Read the model definition and answer for the solid it produces. Units are mm, in the model's axes. Face numbers are marked on the shaded views. Give positions to 0.01 mm unless a question says otherwise; leave off trailing zeros. Loops run counter-clockwise (first coordinate to the right, second up) from the corner with the lowest first, then second, coordinate; pieces in that order, holes last. Notation, with made-up numbers: (20.25, 18.25) -> (66.25, 18.25) arc R12 cw to (66.25, 31.25) -> close; hole circle Ø11 at (3.5, 25). An arc over 180 degrees is marked (long way). One line per item, written item: value. Start each with the question number.
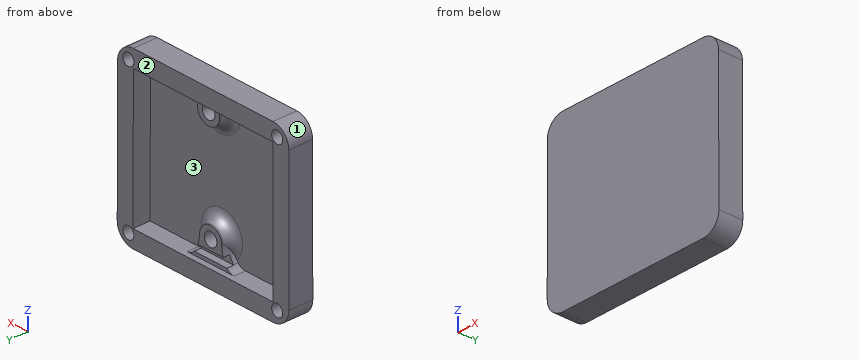
from build123d import *

# Parameters (mm, degrees)
CROQUIS1_R              = 1.3
SALIENTE_EXTRUIR1_DEPTH = 5
VACIADO1_START          = -5
VACIADO1_DEPTH          = 5
VACIADO1_2_OUTLINE_R    = 1.3
VACIADO1_2_DEPTH        = 5
VACIADO1_3_OUTLINE_R    = 1.3
VACIADO1_3_DEPTH        = 5
SALIENTE_EXTRUIR2_START = -1.65
CROQUIS2_R              = 3.5
CROQUIS2_R_2            = 2
SALIENTE_EXTRUIR2_DEPTH = 3.35
CROQUIS3_R              = 2
CORTAR_EXTRUIR1_DEPTH   = 5
REDONDEO1_R             = 5
CROQUIS4_R              = 1.75
CORTAR_EXTRUIR2_DEPTH   = 4
REDONDEO2_R             = 3
CROQUIS5_W              = 10.71017297
CROQUIS5_H              = 2.16113269
CORTAR_EXTRUIR3_DEPTH   = 2
REDONDEO3_R             = 5
CROQUIS6_W              = 134.393326308
CROQUIS6_H              = 117.100902836
CORTAR_EXTRUIR4_DEPTH   = 3


# Read off the part's stored shape, not the designer's step: Vaciado1
with BuildPart() as part:
    # Croquis1 → Saliente-Extruir1 (new body)
    with BuildSketch(Plane(origin=(0, 0, 0), x_dir=(1, 0, 0), z_dir=(0, 1, 0))):
        Polygon((-21.910650365, -18.655769069), (22.326249635, -18.714369069), (22.443043136, 20.685314639), (-21.956956864, 20.744230931), align=None)
        with Locations(Location((0.268043136, -16.390769069, 0), (0, 0, 270))):
            Circle(CROQUIS1_R, mode=Mode.SUBTRACT)
        with Locations(Location((-0.366956864, 14.724230931, 0), (0, 0, 270))):
            Circle(CROQUIS1_R, mode=Mode.SUBTRACT)
    extrude(amount=SALIENTE_EXTRUIR1_DEPTH)

    # Vaciado1 outline → Vaciado1 (add)
    with BuildSketch(Plane(origin=(0, 0, 0), x_dir=(1, 0, 0), z_dir=(0, 1, 0)).offset(VACIADO1_START)):
        Polygon((-26.904785129, -23.649157796), (27.311430385, -23.720977255), (27.457867021, 25.678664653), (-26.962844589, 25.750877863), align=None)
    extrude(amount=VACIADO1_DEPTH)

    # Vaciado1 2 outline → Vaciado1 2 (add)
    # profile 1 of 3: a face of its own
    with BuildSketch(Plane(origin=(0, 0, 0), x_dir=(1, 0, 0), z_dir=(0, 1, 0))):
        Polygon((-26.904785129, -23.649157796), (27.311430385, -23.720977255), (27.457867021, 25.678664653), (-26.962844589, 25.750877863), align=None)
        Polygon((22.443043136, 20.685314639), (22.326249635, -18.714369069), (-21.910650365, -18.655769069), (-21.956956864, 20.744230931), align=None, mode=Mode.SUBTRACT)
    # profile 2 of 3: a face of its own
    with BuildSketch(Plane(origin=(0, 0, 0), x_dir=(1, 0, 0), z_dir=(0, 1, 0))):
        with Locations((0.268043136, -16.390769069)):
            Circle(VACIADO1_2_OUTLINE_R)
    # profile 3 of 3: a face of its own
    with BuildSketch(Plane(origin=(0, 0, 0), x_dir=(1, 0, 0), z_dir=(0, 1, 0))):
        with Locations((-0.366956864, 14.724230931)):
            Circle(VACIADO1_2_OUTLINE_R)
    extrude(amount=VACIADO1_2_DEPTH)

    # Vaciado1 3 outline → Vaciado1 3 (cut)
    with BuildSketch(Plane(origin=(0, 0, 0), x_dir=(1, 0, 0), z_dir=(0, 1, 0))):
        Polygon((-21.910650365, -18.655769069), (22.326249635, -18.714369069), (22.443043136, 20.685314639), (-21.956956864, 20.744230931), align=None)
        with Locations((0.268043136, -16.390769069)):
            Circle(VACIADO1_3_OUTLINE_R, mode=Mode.SUBTRACT)
        with Locations((-0.366956864, 14.724230931)):
            Circle(VACIADO1_3_OUTLINE_R, mode=Mode.SUBTRACT)
    extrude(amount=VACIADO1_3_DEPTH, mode=Mode.SUBTRACT)

    # Croquis2 → Saliente-Extruir2 (add)
    # profile 1 of 2: a face of its own
    with BuildSketch(Plane(origin=(0, 5, 0), x_dir=(1, 0, 0), z_dir=(0, 1, 0)).offset(SALIENTE_EXTRUIR2_START)):
        with Locations((0.268043136, -16.390769069)):
            Circle(CROQUIS2_R)
        with Locations(Location((0.268043136, -16.390769069, 0), (0, 0, 270))):
            Circle(CROQUIS2_R_2, mode=Mode.SUBTRACT)
    # profile 2 of 2: a face of its own
    with BuildSketch(Plane(origin=(0, 5, 0), x_dir=(1, 0, 0), z_dir=(0, 1, 0)).offset(SALIENTE_EXTRUIR2_START)):
        with BuildLine():
            Line((-6.64056044, 20.723906938), (5.906646712, 20.723906938))
            add(Edge.make_bspline(
                [(3.133043136, 14.724230931), (3.271851145, 18.789959359), (5.906646712, 20.723906938)],
                knots=[0, 0, 0, 0.918206359, 0.918206359, 0.918206359], degree=2))
            ThreePointArc((3.133043136, 14.724230931), (-0.366956864, 11.224230931), (-3.866956864, 14.724230931))
            add(Edge.make_bspline(
                [(-3.866956864, 14.724230931), (-4.005764873, 18.789959359), (-6.64056044, 20.723906938)],
                knots=[0, 0, 0, 0.918206359, 0.918206359, 0.918206359], degree=2))
        make_face()
        with Locations(Location((-0.366956864, 14.724230931, 0), (0, 0, 270))):
            Circle(CROQUIS2_R_2, mode=Mode.SUBTRACT)
    extrude(amount=-SALIENTE_EXTRUIR2_DEPTH)

    # Croquis3 → Cortar-Extruir1 (cut)
    with BuildSketch(Plane(origin=(0, 5, 0), x_dir=(1, 0, 0), z_dir=(0, 1, 0))):
        with Locations(Location((-0.366956864, 14.724230931, 0), (0, 0, 270))):
            Circle(CROQUIS3_R)
        with Locations(Location((0.268043136, -16.390769069, 0), (0, 0, 270))):
            Circle(CROQUIS3_R)
    extrude(amount=-CORTAR_EXTRUIR1_DEPTH, mode=Mode.SUBTRACT)

    # Redondeo1
    redondeo1_edges = [part.edges().sort_by_distance(p)[0] for p in [
        (-26.962844589, 0, -25.750877863),
        (27.457867021, 0, -25.678664653),
    ]]
    fillet(redondeo1_edges, radius=REDONDEO1_R)

    # Croquis4 → Cortar-Extruir2 (cut)
    with BuildSketch(Plane(origin=(0, 5, 0), x_dir=(1, 0, 0), z_dir=(0, 1, 0))):
        with Locations(Location((-23.233010561, -20.350621098, 0), (0, 0, 270))):
            Circle(CROQUIS4_R)
        with Locations(Location((23.918815335, -20.350621098, 0), (0, 0, 270))):
            Circle(CROQUIS4_R)
        with Locations(Location((23.918815335, 22.291734245, 0), (0, 0, 270))):
            Circle(CROQUIS4_R)
        with Locations(Location((-23.233010561, 22.291734245, 0), (0, 0, 270))):
            Circle(CROQUIS4_R)
    extrude(amount=-CORTAR_EXTRUIR2_DEPTH, mode=Mode.SUBTRACT)

    # Redondeo2
    # the kernel refuses this fillet: 3 mm, written as the material it adds along each edge
    with BuildSketch(Plane(origin=(0.268043136, 0, 16.390769069), x_dir=(-0.004466262982364763, 0, 0.9999900261977478), z_dir=(0.9999900261977478, 0, 0.004466262982364763))) as redondeo2_piece_1_section:
        with BuildLine():
            CenterArc((3.5 + REDONDEO2_R, -REDONDEO2_R), REDONDEO2_R, 90, 90)
            Line((3.5, -REDONDEO2_R), (3.5 - REDONDEO2_R * 0.02, -REDONDEO2_R))
            Line((3.5 - REDONDEO2_R * 0.02, -REDONDEO2_R), (3.5 - REDONDEO2_R * 0.02, REDONDEO2_R * 0.02))
            Line((3.5 - REDONDEO2_R * 0.02, REDONDEO2_R * 0.02), (3.5 + REDONDEO2_R, REDONDEO2_R * 0.02))
            Line((3.5 + REDONDEO2_R, REDONDEO2_R * 0.02), (3.5 + REDONDEO2_R, 0))
        make_face()
    redondeo2_piece_1 = revolve(axis=Axis((0.268043136, 0, 16.390769069), (0, -1, 0)), revolution_arc=359.64, mode=Mode.PRIVATE)
    redondeo2_piece_1 = split(redondeo2_piece_1, bisect_by=Plane(origin=(0.265003809, 0.854230432, 18.685144847), z_dir=(0.0013246847899521655, 0, -0.9999991226047188)), keep=Keep.TOP, mode=Mode.PRIVATE)
    add(redondeo2_piece_1)
    with BuildSketch(Plane(origin=(-0.366956864, 0, -14.724230931), x_dir=(0.003141587485879655, 0, -0.9999950652018582), z_dir=(-0.9999950652018582, 0, -0.003141587485879655))) as redondeo2_piece_2:
        with BuildLine():
            CenterArc((3.5 + REDONDEO2_R, -REDONDEO2_R), REDONDEO2_R, 90, 90)
            Line((3.5, -REDONDEO2_R), (3.5 - REDONDEO2_R * 0.02, -REDONDEO2_R))
            Line((3.5 - REDONDEO2_R * 0.02, -REDONDEO2_R), (3.5 - REDONDEO2_R * 0.02, REDONDEO2_R * 0.02))
            Line((3.5 - REDONDEO2_R * 0.02, REDONDEO2_R * 0.02), (3.5 + REDONDEO2_R, REDONDEO2_R * 0.02))
            Line((3.5 + REDONDEO2_R, REDONDEO2_R * 0.02), (3.5 + REDONDEO2_R, 0))
        make_face()
    revolve(axis=Axis((-0.366956864, 0, -14.724230931), (0, -1, 0)), revolution_arc=359.64)
    with BuildSketch(Plane(origin=(5.884103635, 0, -20.707287416), x_dir=(0.9999991196116186, -2.6407019803235333e-15, 0.001326942345288348), z_dir=(0, 1, 0))) as redondeo2_piece_3:
        with BuildLine():
            CenterArc((1.172300158, -3), REDONDEO2_R, 90, 51.414502479)
            Line((-1.172734926, -1.128954716), (-1.219635628, -1.09153381))
            ThreePointArc((-1.219635628, -1.09153381), (-0.664607818, -0.483065198), (-0.035769429, 0.048172066))
            Line((-0.035769429, 0.048172066), (0, 0.06))
            Line((0, 0.06), (1.172300158, 0.06))
            Line((1.172300158, 0.06), (1.172300158, 0))
        make_face()
    extrude(amount=3.35)
    with BuildSketch(Plane(origin=(-6.64056044, 3.35, -20.723906938), x_dir=(-0.9999991196114262, 0, -0.0013269424902280428), z_dir=(0, -1, 0))) as redondeo2_piece_4:
        with BuildLine():
            CenterArc((1.1576947, -3), REDONDEO2_R, 89.999999992, 50.80553693)
            Line((-1.167321988, -1.104136767), (-1.213822322, -1.066219502))
            ThreePointArc((-1.213822322, -1.066219502), (-0.660180294, -0.471028769), (-0.035438663, 0.048415919))
            Line((-0.035438663, 0.048415919), (0, 0.06))
            Line((0, 0.06), (1.157694701, 0.06))
            Line((1.157694701, 0.06), (1.157694701, 0))
        make_face()
    extrude(amount=3.35)

    # Croquis5 → Cortar-Extruir3 (cut)
    with BuildSketch(Plane(origin=(0, 3.35, 0), x_dir=(1, 0, 0), z_dir=(0, 1, 0))):
        with Locations((-0.296000529, 18.628716842)):
            Rectangle(CROQUIS5_W, CROQUIS5_H)
    extrude(amount=-CORTAR_EXTRUIR3_DEPTH, mode=Mode.SUBTRACT)

    # Redondeo3
    redondeo3_edges = [part.edges().sort_by_distance(p)[0] for p in [
        (-26.904785129, 0, 23.649157796),
        (27.311430385, 0, 23.720977255),
    ]]
    fillet(redondeo3_edges, radius=REDONDEO3_R)

    # Croquis6 → Cortar-Extruir4 (cut)
    with BuildSketch(Plane.XZ.offset(5)):
        with Locations((-0.420435638, 0)):
            Rectangle(CROQUIS6_W, CROQUIS6_H)
    extrude(amount=-CORTAR_EXTRUIR4_DEPTH, mode=Mode.SUBTRACT)


solid = part.part
Item 1: Section C-C, the plane x = 9.5 is taken. Determine the outline of the cut face in (y, z).
Item 2: Flat-ended cylindrical pins translate along their axes: pin 1 (4.5 mm diameter, centred on x = -0.5, z = -15.5, fed in from +Y); pin 2 (4 mm diameter, centred on y = 1, z = -6, fed in from +X); pin 3 (2 mm diameter, centred on x = -9.5, y = 1.5, fed in from +Z). Find the tip coordinate at first contact, or state that the pin passes through.
Item 3: Consider L1, parallel to X at y = 3.75, z = -15.5; L2, parallel to Z at x = 15.5, y = 4.25; L3, parallel to Z at x = -22, y = 4.75. Determine where each line is inside the solid, lowest interval first. Write a range as [from, to].
Item 4: Determine the mould class of the marked faces 1, 2 and 3 for opening direction Z: pulls with the +Z half, pulls with the -Z half, needs draft (parallel to the pull), parting line crosses it, or undercut.
Item 5: Section B-B, the plane z = 20.5 is taken. Determine the outline of the cut face in (x, y), plus the area to 3 significant figures.
Item 6: Section A-A, the plane y = 4 is taken. Determine the outline of the cut face in (x, z).
Computed values:
1. outline: (-2, -25.7) -> (5, -25.7) -> (5, -20.7) -> (0, -20.7) -> (0, 18.7) -> (5, 18.7) -> (5, 23.7) -> (-2, 23.7) -> close
2. pin 1: y = 3.35
2. pin 2: x = 27.41
2. pin 3: z = 23.67
3. L1: [-26.95, -21.95], [22.43, 27.43]
3. L2: [-25.69, -20.69], [18.71, 23.71]
3. L3: [-25.74, -23.53], [-21.05, 19.11], [21.59, 23.65]
4. face 1: pulls with the +Z half
4. face 2: needs draft
4. face 3: undercut
5. outline: (-26.56, -2) -> (27, -2) -> (27, 5) -> (25.66, 5) -> (25.66, 1) -> (22.18, 1) -> (22.18, 5) -> (-21.49, 5) -> (-21.49, 1) -> (-24.98, 1) -> (-24.98, 5) -> (-26.56, 5) -> close
5. area: 347 mm²
6. outline: (-26.96, -20.74) arc R5 ccw to (-21.95, -25.74) -> (22.45, -25.69) arc R5 ccw to (27.44, -20.67) -> (27.33, 18.73) arc R5 ccw to (22.32, 23.71) -> (-21.92, 23.66) arc R5 ccw to (-26.91, 18.66) -> close; hole circle Ø3.5 at (-23.23, -22.29); hole circle Ø3.5 at (-23.23, 20.35); hole (-21.96, -20.74) -> (22.44, -20.69) -> (22.33, 18.71) -> (-21.91, 18.66) -> close; hole circle Ø3.5 at (23.92, -22.29); hole circle Ø3.5 at (23.92, 20.35)
